Read the model definition and answer for the solid it produces. Units are mm, in the model's axes. A direction names the side the tool comes from. Coordinates: 2 decimals unless noted, no trailing zeros. Write each loop counter-clockwise with the first axis right and the second up, starting at its lowest first coordinate (ties: lowest second). Pieces come first, ordered by that corner, then holes.
Item 1: Section C-C (z = -13) is taken. Give the vertices of the cut face in (x, y), then the cut area to 3 significant figures.
Item 2: Straight lines are drawn through the part: probe 1 along X at (y, z) = (37, -3.4); probe 2 along Y at (x, z) = (6.75, -4.2); probe 3 along Y at (x, z) = (43.5, -4.75). For each, find the intervals that lie inside material, in ascending order.
Item 3: Section D-D (x = 34) is taken. Give the vertices of the cut face in (y, z).
Item 4: Section A-A (x = 14) is taken. Give the vertices of the cut face in (y, z), then the cut area to 3 significant figures.
Item 5: Determine the mould class of faces 5 (the face through (15.5, 48, -2)), 6 (the face through (47, 30, -4)), 7 (the face through (28, 0, -8)) for opening direction Y: released by +Y, released by -Y, zero draft, split by the parting line, or undercut.
Item 6: Each of these flat-tipped pins is pushed along its axis until it touches: P1, Ø10, axis at x = 47, y = 37.5, coming from the -Z side; P2, Ø3.5, axis at x = 53.5, z = -10.5, coming from the -Y side; P3, Ø4, axis at y = 33, z = 3.5, coming from the +X side; P4, Ø1.5, axis at x = 21, y = 34, coming from the +Z side. Where does it stop, or does it pass through?
Item 7: Section B-B (y = 30.5) is taken. Give the vertices of the cut face in (x, z).
Item 8: A tool of negligible diameter and unlimited length cuts with its end or side. For faces 1 (the face through (45, 30, -2.5)), 2 (the face through (49, 24, 4)), 3 (the face through (26, 5, 0.4)), 4 (the face through (40.5, 49, -2)), from which of +Z, -Z, +X, -X, +Y, -Y can it reach the whole face along a straight path? Write none if from no direction.
from build123d import *

# Parameters (mm, degrees)
BOSS_EXTRUDE1_OUTLINE_W      = 4.95
BOSS_EXTRUDE1_OUTLINE_H      = 2.9
BOSS_EXTRUDE1_DEPTH          = 51
BOSS_EXTRUDE1_2_OUTLINE_W    = 46.1
BOSS_EXTRUDE1_2_OUTLINE_H    = 2.9
BOSS_EXTRUDE1_2_DEPTH        = 6
SKETCH2_W                    = 56
SKETCH2_H                    = 51
SKETCH2_W_2                  = 42
SKETCH2_H_2                  = 32
BOSS_EXTRUDE2_DEPTH          = 2.5
BOSS_EXTRUDE3_DEPTH          = 5
M3X0_5_TAPPED_HOLE1_D        = 2.5
M3X0_5_TAPPED_HOLE1_DEPTH    = 4
M3X0_5_TAPPED_HOLE1_TIP      = 0.751075774
SKETCH9_W                    = 56
SKETCH9_H                    = 2.5
BOSS_EXTRUDE4_DEPTH          = 5
SKETCH9_3_W                  = 56
SKETCH9_3_H                  = 9.5
BOSS_EXTRUDE5_DEPTH          = 2.5
M2_5X0_45_TAPPED_HOLE1_D     = 2.05
M2_5X0_45_TAPPED_HOLE1_DEPTH = 6.35
M2_5X0_45_TAPPED_HOLE1_TIP   = 0.615882135
BOSS_EXTRUDE6_REACH          = 78.688
SKETCH12_W                   = 4
SKETCH12_H                   = 51
SKETCH13_W                   = 4
SKETCH13_H                   = 9
CUT_EXTRUDE1_DEPTH           = 2.5
SKETCH14_W                   = 12
SKETCH14_H                   = 30
CUT_EXTRUDE2_DEPTH           = 3
CUT_EXTRUDE3_DEPTH           = 78.62731478
SKETCH17_W                   = 5
SKETCH17_H                   = 51
CUT_EXTRUDE4_DEPTH           = 3
SKETCH18_W                   = 5
SKETCH18_H                   = 51
CUT_EXTRUDE5_DEPTH           = 3
FILLET1_R                    = 3
MOVE_FACE1_BY                = 0.2
MOVE_FACE1_2_BY              = 0.2
MOVE_FACE1_3_BY              = 0.2
MOVE_FACE1_4_BY              = 0.2
MOVE_FACE1_5_BY              = 0.2
MOVE_FACE1_6_BY              = 0.2
MOVE_FACE1_7_BY              = 0.2
MOVE_FACE1_8_BY              = 0.2
MOVE_FACE1_9_BY              = 0.2
MOVE_FACE1_10_BY             = 0.2
MOVE_START                   = 4.55
MOVE_FACE2_OUTLINE_W         = 45
MOVE_FACE2_OUTLINE_H         = 2.9
MOVE_FACE2_DEPTH             = 46.9


# Read off the part's stored shape, not the designer's step: Boss-Extrude1, Move Face2
with BuildPart() as part:
    # Boss-Extrude1 outline → Boss-Extrude1 (new body)
    with BuildSketch(Plane(origin=(0, 0, 0), x_dir=(1, 0, 0), z_dir=(0, 1, 0))):
        with Locations((2.475, -1.45)):
            Rectangle(BOSS_EXTRUDE1_OUTLINE_W, BOSS_EXTRUDE1_OUTLINE_H)
        with Locations((53.525, -1.45)):
            Rectangle(BOSS_EXTRUDE1_OUTLINE_W, BOSS_EXTRUDE1_OUTLINE_H)
    extrude(amount=BOSS_EXTRUDE1_DEPTH)

    # Boss-Extrude1 2 outline → Boss-Extrude1 2 (add)
    with BuildSketch(Plane(origin=(0, 0, 0), x_dir=(1, 0, 0), z_dir=(0, 1, 0))):
        with Locations((28, -1.45)):
            Rectangle(BOSS_EXTRUDE1_2_OUTLINE_W, BOSS_EXTRUDE1_2_OUTLINE_H)
    extrude(amount=BOSS_EXTRUDE1_2_DEPTH)

    # Sketch2 → Boss-Extrude2 (add)
    with BuildSketch(Plane.XY.offset(2.9)):
        with Locations((28, 25.5)):
            Rectangle(SKETCH2_W, SKETCH2_H)
        with Locations((28, 24.54)):
            Rectangle(SKETCH2_W_2, SKETCH2_H_2, mode=Mode.SUBTRACT)
    extrude(amount=BOSS_EXTRUDE2_DEPTH)

    # Sketch3 → Boss-Extrude3 (add)
    with BuildSketch(Plane(origin=(0, 0, 0), x_dir=(-1, 0, 0), z_dir=(0, 0, -1))):
        Polygon((-56, 51), (-40.5, 51), (-40.5, 46), (-15.5, 46), (-15.5, 51), (0, 51), (0, 0), (-56, 0), align=None)
    extrude(amount=BOSS_EXTRUDE3_DEPTH)

    # M3x0.5 Tapped Hole1
    with Locations(Plane(origin=(0, 0, -5), x_dir=(-1, 0, 0), z_dir=(0, 0, -1))):
        with Locations((-49.25, 37), (-6.75, 37), (-6.75, 10), (-49.25, 10)):
            Hole(M3X0_5_TAPPED_HOLE1_D / 2, depth=M3X0_5_TAPPED_HOLE1_DEPTH)
            with Locations((0, 0, -(M3X0_5_TAPPED_HOLE1_DEPTH + M3X0_5_TAPPED_HOLE1_TIP / 2))):  # 118° drill point
                Cone(0, M3X0_5_TAPPED_HOLE1_D / 2, M3X0_5_TAPPED_HOLE1_TIP, mode=Mode.SUBTRACT)



with BuildPart() as body_2:
    # Sketch9 → Boss-Extrude4 (new body)
    with BuildSketch(Plane.XZ):
        with Locations((28, -15.75)):
            Rectangle(SKETCH9_W, SKETCH9_H)
    extrude(amount=-BOSS_EXTRUDE4_DEPTH)


with BuildPart() as part_1:
    add(part.part)

    add(body_2.part)  # Boss-Extrude5 merges body 2
    # Sketch9<3> → Boss-Extrude5 (add)
    with BuildSketch(Plane.XZ):
        with Locations((28, -9.75)):
            Rectangle(SKETCH9_3_W, SKETCH9_3_H)
    extrude(amount=-BOSS_EXTRUDE5_DEPTH)

    # M2.5x0.45 Tapped Hole1
    with Locations(Plane(origin=(0, 51, 0), x_dir=(1, 0, 0), z_dir=(0, 1, 0))):
        with Locations((4, 2.1), (52, 2.1)):
            Hole(M2_5X0_45_TAPPED_HOLE1_D / 2, depth=M2_5X0_45_TAPPED_HOLE1_DEPTH)
            with Locations((0, 0, -(M2_5X0_45_TAPPED_HOLE1_DEPTH + M2_5X0_45_TAPPED_HOLE1_TIP / 2))):  # 118° drill point
                Cone(0, M2_5X0_45_TAPPED_HOLE1_D / 2, M2_5X0_45_TAPPED_HOLE1_TIP, mode=Mode.SUBTRACT)

    # Boss-Extrude6: up to this face of the body (flat: up to its plane)
    boss_extrude6_end = Plane(part_1.part.faces().sort_by_distance((28, 2.5, -17))[0])
    # Sketch12 → Boss-Extrude6 (add, up to the picked face)
    with BuildSketch(Plane(origin=(0, 0, -5), x_dir=(-1, 0, 0), z_dir=(0, 0, -1)), mode=Mode.PRIVATE) as boss_extrude6_sk1:
        with Locations((-2, 25.5)):
            Rectangle(SKETCH12_W, SKETCH12_H)
    boss_extrude6_tool1 = split(extrude(boss_extrude6_sk1.sketch, amount=BOSS_EXTRUDE6_REACH, mode=Mode.PRIVATE), bisect_by=boss_extrude6_end, keep=Keep.BOTH, mode=Mode.PRIVATE)
    # Sketch12 → Boss-Extrude6 (add, up to the picked face)
    with BuildSketch(Plane(origin=(0, 0, -5), x_dir=(-1, 0, 0), z_dir=(0, 0, -1)), mode=Mode.PRIVATE) as boss_extrude6_sk2:
        with Locations((-54, 25.5)):
            Rectangle(SKETCH12_W, SKETCH12_H)
    boss_extrude6_tool2 = split(extrude(boss_extrude6_sk2.sketch, amount=BOSS_EXTRUDE6_REACH, mode=Mode.PRIVATE), bisect_by=boss_extrude6_end, keep=Keep.BOTH, mode=Mode.PRIVATE)
    add(boss_extrude6_tool1.solids().sort_by(Axis((2, 25.5, -5), (0, 0, -1)))[0])
    add(boss_extrude6_tool2.solids().sort_by(Axis((54, 25.5, -5), (0, 0, -1)))[0])

    # Sketch13 → Cut-Extrude1 (cut)
    with BuildSketch(Plane(origin=(0, 0, -5), x_dir=(-1, 0, 0), z_dir=(0, 0, -1))):
        with Locations((-45, 30)):
            Rectangle(SKETCH13_W, SKETCH13_H)
    extrude(amount=-CUT_EXTRUDE1_DEPTH, mode=Mode.SUBTRACT)

    # Sketch14 → Cut-Extrude2 (cut)
    with BuildSketch(Plane.ZY.offset(-52)):
        with Locations((-11, 31)):
            Rectangle(SKETCH14_W, SKETCH14_H)
    extrude(amount=-CUT_EXTRUDE2_DEPTH, mode=Mode.SUBTRACT)

    # Sketch15 → Cut-Extrude3 (cut, through all)
    with BuildSketch(Plane.ZY):
        Polygon((5.4, 0), (0.4, 0), (0.4, 5), (2.9, 5), (2.9, 2.5), (5.4, 2.5), align=None)
    extrude(amount=-CUT_EXTRUDE3_DEPTH, mode=Mode.SUBTRACT)

    # Sketch17 → Cut-Extrude4 (cut)
    with BuildSketch(Plane.ZY):
        with Locations((2.9, 25.5)):
            Rectangle(SKETCH17_W, SKETCH17_H)
    extrude(amount=-CUT_EXTRUDE4_DEPTH, mode=Mode.SUBTRACT)

    # Sketch18 → Cut-Extrude5 (cut)
    with BuildSketch(Plane(origin=(56, 0, 0), x_dir=(0, 0, -1), z_dir=(1, 0, 0))):
        with Locations((-2.9, 25.5)):
            Rectangle(SKETCH18_W, SKETCH18_H)
    extrude(amount=-CUT_EXTRUDE5_DEPTH, mode=Mode.SUBTRACT)

    # Fillet1
    fillet1_edges = [part_1.edges().sort_by_distance(p)[0] for p in [
        (56, 0, -8.3),
        (0, 0, -8.3),
    ]]
    fillet(fillet1_edges, radius=FILLET1_R)

    # Move Face1: a face moved inward by 0.2
    extrude(part_1.faces().sort_by_distance((28, 3.75, 2.9))[0], amount=MOVE_FACE1_BY, dir=(0, 0, 1), mode=Mode.SUBTRACT)

    # Move Face1 2: a face moved inward by 0.2
    extrude(part_1.faces().sort_by_distance((28, 2.5, 4.15))[0], amount=MOVE_FACE1_2_BY, dir=(0, 1, 0), mode=Mode.SUBTRACT)

    # Move Face1 3: a face moved inward by 0.2
    extrude(part_1.faces().sort_by_distance((28, 5, 1.65))[0], amount=MOVE_FACE1_3_BY, dir=(0, 1, 0), mode=Mode.SUBTRACT)

    # Move Face1 4: a face moved inward by 0.2
    extrude(part_1.faces().sort_by_distance((3, 27.358465608, 2.933068783))[0], amount=MOVE_FACE1_4_BY, dir=(1, 0, 0), mode=Mode.SUBTRACT)

    # Move Face1 5: a face moved inward by 0.2
    extrude(part_1.faces().sort_by_distance((53, 27.358465608, 2.933068783))[0], amount=MOVE_FACE1_5_BY, dir=(-1, 0, 0), mode=Mode.SUBTRACT)

    # Move Face1 6: a face moved inward by 0.2
    extrude(part_1.faces().sort_by_distance((28, 2.5, -9.75))[0], amount=MOVE_FACE1_6_BY, dir=(0, -1, 0), mode=Mode.SUBTRACT)

    # Move Face1 7: a face moved inward by 0.2
    extrude(part_1.faces().sort_by_distance((28, 3.75, -14.5))[0], amount=MOVE_FACE1_7_BY, dir=(0, 0, -1), mode=Mode.SUBTRACT)

    # Move Face1 8: a face moved inward by 0.2
    extrude(part_1.faces().sort_by_distance((28, 5, -15.75))[0], amount=MOVE_FACE1_8_BY, dir=(0, -1, 0), mode=Mode.SUBTRACT)

    # Move Face1 9: a face moved inward by 0.2
    extrude(part_1.faces().sort_by_distance((4, 26.999674338, -10.948436822))[0], amount=MOVE_FACE1_9_BY, dir=(-1, 0, 0), mode=Mode.SUBTRACT)

    # Move Face1 10: a face moved inward by 0.2
    extrude(part_1.faces().sort_by_distance((52, 9.47070626, -10.809390048))[0], amount=MOVE_FACE1_10_BY, dir=(1, 0, 0), mode=Mode.SUBTRACT)

    # Move Face2 outline → Move Face2 (cut)
    with BuildSketch(Plane.YZ.offset(MOVE_START)):
        with Locations((28.5, 1.45)):
            Rectangle(MOVE_FACE2_OUTLINE_W, MOVE_FACE2_OUTLINE_H)
    extrude(amount=MOVE_FACE2_DEPTH, mode=Mode.SUBTRACT)


solid = part_1.part
Established:
1. outline: (0, 3) arc R3 ccw to (3, 0) - (53, 0) arc R3 ccw to (56, 3) - (56, 51) - (52, 51) - (52, 46) - (55, 46) - (55, 16) - (52.2, 16) - (52.2, 2.3) - (3.8, 2.3) - (3.8, 51) - (0, 51) - close
1. area: 412 mm2
2. probe 1: x = 0 to 5.5, 8 to 48, 50.5 to 56
2. probe 2: y = 0 to 8.75, 11.25 to 35.75, 38.25 to 51
2. probe 3: y = 0 to 25.5, 34.5 to 51
3. outline: (0, -17) - (4.8, -17) - (4.8, -14.7) - (2.3, -14.7) - (2.3, -5) - (46, -5) - (46, 0) - (6, 0) - (6, 2.9) - (8.54, 2.9) - (8.54, 5.4) - (2.7, 5.4) - (2.7, 3.1) - (5.2, 3.1) - (5.2, 0.4) - (0, 0.4) - close; (40.54, 2.9) - (51, 2.9) - (51, 5.4) - (40.54, 5.4) - close
4. outline: (0, -17) - (4.8, -17) - (4.8, -14.7) - (2.3, -14.7) - (2.3, -5) - (51, -5) - (51, 0) - (6, 0) - (6, 2.9) - (8.54, 2.9) - (8.54, 5.4) - (2.7, 5.4) - (2.7, 3.1) - (5.2, 3.1) - (5.2, 0.4) - (0, 0.4) - close; (40.54, 2.9) - (51, 2.9) - (51, 5.4) - (40.54, 5.4) - close
4. area: 333 mm2
5. face 5: zero draft
5. face 6: undercut
5. face 7: released by -Y
6. P1: stops at z = -5
6. P2: stops at y = 0
6. P3: stops at x = 52.8
6. P4: stops at z = 0
7. outline: (0, -17) - (3.8, -17) - (3.8, -5) - (43, -5) - (43, -2.5) - (47, -2.5) - (47, -5) - (55, -5) - (55, -17) - (56, -17) - (56, 0.4) - (52.8, 0.4) - (52.8, 5.4) - (49, 5.4) - (49, 2.9) - (51.45, 2.9) - (51.45, 0) - (4.55, 0) - (4.55, 2.9) - (7, 2.9) - (7, 5.4) - (3.2, 5.4) - (3.2, 0.4) - (0, 0.4) - close
8. face 1: -Z
8. face 2: +Z
8. face 3: -Y
8. face 4: -Z, +Y
